Build history of the part. All positions in model axes, mm. A direction names the side the tool comes from. Give positions to 0.01 mm unless a question says otherwise; leave off trailing zeros. Order: outer loops, then holes, each group sorted by start corner. A loop starts at its lowest first (then second) coordinate and runs counter-clockwise, first axis right, second up. Notation, with made-up numbers: (13, -32.5) -> (32, -32.5) arc R30 ccw to (32, 3.5) -> close; hole circle Ø5 at (40.25, -20). An arc over 180 degrees is marked (long way). One line per item, written item: value. Start each with the question number.
(1) Which spindle directions (+Z, -Z, +X, -X, +Y, -Y) get a long thin tool onto all of the face, cutting with end or side? Do faces 4 (the cylindrical face through (15.958, 19.524, -4.336)), 5 (the flat face through (13, 15, -9)). Say none if no direction does.
(2) Saw through at C-C on x = 17. Give the cut face in (y, z).
(3) Pin check, flat tips, straight feed: pin 1 (1 mm diameter, centred on x = 15.5, y = 11.5, fed in from -Z); pin 2 (4 mm diameter, centred on y = 2, z = -10, fed in from -X); pin 3 (12 mm diameter, centred on x = 3.5, y = 10.5, fed in from -Z); pin 4 (5 mm diameter, centred on x = 16, z = 11, fed in from -Y). Stop position of each tip, or through.
(4) Probe line 1 (Z direction, x = 14, y = 0); line 2 (Z direction, x = 9, y = 0.5); line 3 (X direction, y = -4, z = -17.5). List the from-to ranges inside material, lowest first.
(5) Saw through at A-A on z = 0. Give the cut face in (x, y).
(6) Two-plate mould, pull along Y, no slides. Class faces 1 (the cylindrical face through (8.944, -14.334, 9.139)), 2 (the cylindrical face through (9.86, 11.99, 0.53)), 3 (the flat face through (20, 12.4, 0.3)): +Y half, -Y half, draft (parallel to the pull), parting line (faces both ways), or undercut.
```python
from build123d import *

# Parameters (mm, degrees)
F2_SIZE  = 1
F3_SIZE2 = 0.437443
F3_SIZE  = 5
F4_R     = 12
F5_DEPTH = 69.3


with BuildPart() as f1:
    # F0 (on Front) → F1 (revolve)
    with BuildSketch(Plane.XZ):
        Polygon((0, 17), (0, 0), (20, 0), (20, 20), (13, 20), (13, 17), align=None)
    revolve(axis=Axis((10, 0, 0), (1, 0, 0)))

    # F2
    f2_edges = [f1.edges().sort_by_distance(p)[0] for p in [
        (20, 0, -20),
    ]]
    chamfer(f2_edges, length=F2_SIZE)

    # F3
    f3_edges = [f1.edges().sort_by_distance(p)[0] for p in [
        (0, 0, -17),
    ]]
    chamfer(f3_edges, length=F3_SIZE, length2=F3_SIZE2)

    # F4 (on face) → F5 (cut)
    with BuildSketch(Plane(origin=(0, 0, 0), x_dir=(0, -1, 0), z_dir=(-1, 0, 0))):
        Circle(F4_R)
    extrude(amount=-F5_DEPTH, mode=Mode.SUBTRACT)


solid = f1.part
```
Results below:
1. face 4: +X, -X
1. face 5: -X
2. outline: circle Ø40 at (0, 0); hole circle Ø24 at (0, 0)
3. pin 1: stops at z = -16.7
3. pin 2: stops at x = 0
3. pin 3: stops at z = -16.34
3. pin 4: stops at y = -18.1
4. line 1: z = -20 to -12, 12 to 20
4. line 2: z = -16.99 to -11.99, 11.99 to 16.99
4. line 3: x = 13 to 20
5. outline: (0, -16.56) -> (5, -17) -> (13, -17) -> (13, -20) -> (19, -20) -> (20, -19) -> (20, -12) -> (0, -12) -> close; (0, 12) -> (20, 12) -> (20, 19) -> (19, 20) -> (13, 20) -> (13, 17) -> (5, 17) -> (0, 16.56) -> close
6. face 1: parting line
6. face 2: undercut
6. face 3: draft
